from build123d import *

# Parameters (mm, degrees)
F0_R     = 3.175
F1_DEPTH = 19.05
F3_DEPTH = 12.7


with BuildPart() as f1:
    # F0 (on Top) → F1 (new body)
    with BuildSketch(Plane.XY):
        Circle(F0_R)
    extrude(amount=-F1_DEPTH)

    # F2 (on Front) → F3 (cut, symmetric)
    with BuildSketch(Plane.XZ):
        Polygon((3.41024, 0.097258), (-3.577343, 0.097258), (-3.577343, -3.126712), (-1.249831, -3.126712), (-0.344881, -5.392152), (0.963141, -1.171422), (1.7667, -3.126712), (3.502352, -3.126712), align=None)
    extrude(amount=F3_DEPTH, both=True, mode=Mode.SUBTRACT)


solid = f1.part
For this review, take the finished solid that the model builds, in its own axes (mm). A direction names the side the tool comes from. Round coordinates to 2 decimals unless told otherwise and drop trailing zeros. Loops run counter-clockwise (first coordinate to the right, second up) from the corner with the lowest first, then second, coordinate; pieces in that order, holes last. Notation, with made-up numbers: (-4, -10.75) - (43, -10.75) arc R30 cw to (43, 22.25) - close; hole circle Ø4 at (73.25, -5). An arc over 180 degrees is marked (long way). Put each result on its own line as item: value. Start each with the question number.
1. Consider section A-A on y = 0. State the section outline as (x, z) points (3 decimals).
2. Consider section B-B on x = -2. State the section outline as (y, z) points.
3. Consider section D-D on y = 1.25. State the section outline as (x, z) points.
4. Mouldability with a two-part tool opening along X and no side actions: class faces 3 (the flat face through (0, 0, -19.05)), 4 (the cylindrical face through (3.03, 0.95, -11.97)), 5 (the flat face through (0.3, -0.04, -3.31)), 6 (the flat face through (1.36, -0.04, -2.14)) as +X half, -X half, draft (parallel to the pull), parting line (faces both ways), or undercut.
5. For faces 1 (the flat face through (-2, 0, -3.127)), 2 (the flat face through (2, 0, -3.127)), list the 3-axis set-ups (+Z, -Z, +X, -X, +Y, -Y) from which the entire face can be reached by the end or side of a thin tool; tool diameter is ignored.
6. For probe 1 along Z at (x, y) = (-2.5, 1); probe 2 along X at (y, z) = (-1.5, -4.5); probe 3 along Y at (x, z) = (-1.25, -10.25), list the stretches that pass through material, from the lowest coordinate up. Write a range as [from, to].
7. Consider section C-C on z = -9.5. State the section outline as (x, y) points (3 decimals), plus the area to 3 significant figures.
8. Insertion check: P1, Ø2, axis at x = -2, z = -16.5, coming from the +Y side; P2, Ø3, axis at y = 2, z = -9.5, coming from the +X side; P3, Ø0.6, axis at x = -2, y = -1, coming from the +Z side; P4, Ø3, axis at y = -0.5, z = -14, coming from the +X side (3 decimals). Each pin has a flat end and moves straight along its axis. Give the tip position at first contact, or say it passes through.
Result sheet:
1. outline: (-3.175, -19.05) - (3.175, -19.05) - (3.175, -3.127) - (1.767, -3.127) - (0.963, -1.171) - (-0.345, -5.392) - (-1.25, -3.127) - (-3.175, -3.127) - close
2. outline: (-2.47, -19.05) - (2.47, -19.05) - (2.47, -3.13) - (-2.47, -3.13) - close
3. outline: (-2.92, -19.05) - (2.92, -19.05) - (2.92, -3.13) - (1.77, -3.13) - (0.96, -1.17) - (-0.34, -5.39) - (-1.25, -3.13) - (-2.92, -3.13) - close
4. face 3: draft
4. face 4: parting line
4. face 5: undercut
4. face 6: +X half
5. face 1: +Z, -X, +Y, -Y
5. face 2: +Z, +X, +Y, -Y
6. probe 1: [-19.05, -3.13]
6. probe 2: [-2.8, -0.7], [-0.07, 2.8]
6. probe 3: [-2.92, 2.92]
7. outline: circle Ø6.35 at (0, 0)
7. area: 31.7 mm^2
8. P1: y = 3.01
8. P2: x = 3.14
8. P3: z = -3.13
8. P4: x = 3.175
